Check sheet for the modelled part. Datum: model origin and axes. Units: mm. A direction names the side the tool comes from. Round coordinates to 2 decimals unless told otherwise and drop trailing zeros. Order: outer loops, then holes, each group sorted by start corner. A loop starts at its lowest first (then second) coordinate and runs counter-clockwise, first axis right, second up.
```python
from build123d import *

# Parameters (mm, degrees)
SKETCH_1_R             = 0.5
EXTRUDE_1_DEPTH        = 8
EXTRUDE_2_DEPTH        = 21.5
EXTRUDE_3_DEPTH        = 9
SKETCH_4_R             = 3
EXTRUDE_4_DEPTH        = 10
EXTRUDE_5_DEPTH        = 9
HOLE_WIZARD_M3_1_D     = 2.5
HOLE_WIZARD_M3_1_DEPTH = 6.5
HOLE_WIZARD_M3_1_TIP   = 0.751075774
SKETCH_10_R            = 11
EXTRUDE_6_DEPTH        = 2
SKETCH_11_R            = 4.75
CUT_EXTRUDE_1_DEPTH    = 22
SKETCH_12_W            = 16
SKETCH_12_H            = 4
EXTRUDE_7_DEPTH        = 20
SKETCH_13_W            = 16
SKETCH_13_H            = 5.5
CUT_EXTRUDE_2_DEPTH    = 4
SKETCH_14_W            = 16
SKETCH_14_H            = 0.410991047
CUT_EXTRUDE_3_DEPTH    = 3
SKETCH_15_W            = 14.932119024
SKETCH_15_H            = 4.421120872
SKETCH_15_W_2          = 1.018591574
SKETCH_15_H_2          = 0.888558607
SKETCH_15_W_3          = 0.910230768
SKETCH_15_W_4          = 1.105280218
SKETCH_15_W_5          = 0.95357509
SKETCH_15_W_6          = 1.365346151
SKETCH_15_W_7          = 14.029885449
SKETCH_15_H_3          = 2.651802524
SKETCH_15_W_8          = 0.733211095
SKETCH_15_H_4          = 0.986717219
SKETCH_15_W_9          = 0.549388278
SKETCH_15_W_10         = 0.68897455
SKETCH_15_W_11         = 1.063804501
SKETCH_15_W_12         = 0.745609389
SKETCH_15_W_13         = 0.832542653
CUT_EXTRUDE_4_DEPTH    = 3
SKETCH_16_W            = 3.5
SKETCH_16_H            = 23
EXTRUDE_8_DEPTH        = 5.5
SKETCH_17_W            = 23
SKETCH_17_H            = 3.5
CUT_EXTRUDE_5_DEPTH    = 1
SKETCH_18_W            = 21.377042826
SKETCH_18_H            = 3.957601196
SKETCH_18_W_2          = 1.139309436
SKETCH_18_H_2          = 1.169291262
SKETCH_18_W_3          = 0.929436644
SKETCH_18_W_4          = 1.109327608
SKETCH_18_W_5          = 1.349182226
SKETCH_18_W_6          = 1.259236744
SKETCH_18_W_7          = 1.319200399
CUT_EXTRUDE_6_DEPTH    = 3


with BuildPart() as part:
    # 草图1 → 凸台-拉伸1 (new body)
    with BuildSketch(Plane(origin=(0, 0, 0), x_dir=(1, 0, 0), z_dir=(0, 1, 0))):
        Polygon((-21, 17.5), (-17.5, 21), (17.5, 21), (21, 17.5), (21, -17.5), (17.5, -21), (-17.5, -21), (-21, -17.5), align=None)
        with Locations(Location((-15.5, 15.5, 0), (0, 0, 270))):
            Circle(SKETCH_1_R, mode=Mode.SUBTRACT)
        with Locations(Location((15.5, 15.5, 0), (0, 0, 270))):
            Circle(SKETCH_1_R, mode=Mode.SUBTRACT)
        with Locations(Location((-15.5, -15.5, 0), (0, 0, 270))):
            Circle(SKETCH_1_R, mode=Mode.SUBTRACT)
        with Locations(Location((15.5, -15.5, 0), (0, 0, 270))):
            Circle(SKETCH_1_R, mode=Mode.SUBTRACT)
    extrude(amount=EXTRUDE_1_DEPTH)

    # 草图2 → 凸台-拉伸2 (add)
    with BuildSketch(Plane.XZ):
        with BuildLine():
            Line((-20.414213562, 14.585786438), (-14.585786438, 20.414213562))
            ThreePointArc((-14.585786438, 20.414213562), (-13.93693974, 20.847759065), (-13.171572875, 21))
            Line((-13.171572875, 21), (13.171572875, 21))
            ThreePointArc((13.171572875, 21), (13.93693974, 20.847759065), (14.585786438, 20.414213562))
            Line((14.585786438, 20.414213562), (20.414213562, 14.585786438))
            ThreePointArc((20.414213562, 14.585786438), (20.847759065, 13.93693974), (21, 13.171572875))
            Line((21, 13.171572875), (21, -13.171572875))
            ThreePointArc((21, -13.171572875), (20.847759065, -13.93693974), (20.414213562, -14.585786438))
            Line((20.414213562, -14.585786438), (14.585786438, -20.414213562))
            ThreePointArc((14.585786438, -20.414213562), (13.93693974, -20.847759065), (13.171572875, -21))
            Line((13.171572875, -21), (-13.171572875, -21))
            ThreePointArc((-13.171572875, -21), (-13.93693974, -20.847759065), (-14.585786438, -20.414213562))
            Line((-14.585786438, -20.414213562), (-20.414213562, -14.585786438))
            ThreePointArc((-20.414213562, -14.585786438), (-20.847759065, -13.93693974), (-21, -13.171572875))
            Line((-21, -13.171572875), (-21, 13.171572875))
            ThreePointArc((-21, 13.171572875), (-20.847759065, 13.93693974), (-20.414213562, 14.585786438))
        make_face()
    extrude(amount=EXTRUDE_2_DEPTH)

    # 草图3 → 凸台-拉伸3 (add)
    with BuildSketch(Plane.XZ.offset(21.5)):
        Polygon((-21, 17.5), (-17.5, 21), (17.5, 21), (21, 17.5), (21, -17.5), (17.5, -21), (-17.5, -21), (-21, -17.5), align=None)
    extrude(amount=EXTRUDE_3_DEPTH)

    # 草图4 → 凸台-拉伸4 (add)
    with BuildSketch(Plane.XZ.offset(30.5)):
        with Locations(Location((-15.5, 15.5, 0), (0, 0, 90))):
            Circle(SKETCH_4_R)
        with Locations(Location((15.5, 15.5, 0), (0, 0, 90))):
            Circle(SKETCH_4_R)
        with Locations(Location((-15.5, -15.5, 0), (0, 0, 90))):
            Circle(SKETCH_4_R)
        with Locations(Location((15.5, -15.5, 0), (0, 0, 90))):
            Circle(SKETCH_4_R)
    extrude(amount=EXTRUDE_4_DEPTH)

    # 草图5 → 凸台-拉伸5 (add)
    with BuildSketch(Plane.XZ.offset(40.5)):
        Polygon((-21, 17.5), (-17.5, 21), (17.5, 21), (21, 17.5), (21, -17.5), (17.5, -21), (-17.5, -21), (-21, -17.5), align=None)
    extrude(amount=-EXTRUDE_5_DEPTH)

    # M3 螺纹孔的螺纹孔钻头1
    with Locations(Plane(origin=(0, 8, 0), x_dir=(1, 0, 0), z_dir=(0, 1, 0))):
        with Locations((-15.5, 15.5), (15.5, 15.5), (-15.5, -15.5), (15.5, -15.5)):
            Hole(HOLE_WIZARD_M3_1_D / 2, depth=HOLE_WIZARD_M3_1_DEPTH)
            with Locations((0, 0, -(HOLE_WIZARD_M3_1_DEPTH + HOLE_WIZARD_M3_1_TIP / 2))):  # 118° drill point
                Cone(0, HOLE_WIZARD_M3_1_D / 2, HOLE_WIZARD_M3_1_TIP, mode=Mode.SUBTRACT)

    # 草图10 → 凸台-拉伸6 (add)
    with BuildSketch(Plane(origin=(0, 8, 0), x_dir=(1, 0, 0), z_dir=(0, 1, 0))):
        with Locations(Location((0, 0, 0), (0, 0, 90))):
            Circle(SKETCH_10_R)
    extrude(amount=EXTRUDE_6_DEPTH)

    # 草图11 → 切除-拉伸1 (cut)
    with BuildSketch(Plane(origin=(0, 10, 0), x_dir=(1, 0, 0), z_dir=(0, 1, 0))):
        with Locations(Location((0, 0, 0), (0, 0, 270))):
            Circle(SKETCH_11_R)
    extrude(amount=-CUT_EXTRUDE_1_DEPTH, mode=Mode.SUBTRACT)

    # 草图12 → 凸台-拉伸7 (add)
    with BuildSketch(Plane.XZ.offset(40.5)):
        with Locations((0, 23)):
            Rectangle(SKETCH_12_W, SKETCH_12_H)
    extrude(amount=-EXTRUDE_7_DEPTH)

    # 草图13 → 切除-拉伸2 (cut)
    with BuildSketch(Plane.XY.offset(25)):
        with Locations((0, -33.25)):
            Rectangle(SKETCH_13_W, SKETCH_13_H)
    extrude(amount=-CUT_EXTRUDE_2_DEPTH, mode=Mode.SUBTRACT)

    # 草图14 → 切除-拉伸3 (cut)
    with BuildSketch(Plane.XY.offset(25)):
        with Locations((0, -28.356047823)):
            Rectangle(SKETCH_14_W, SKETCH_14_H)
    extrude(amount=-CUT_EXTRUDE_3_DEPTH, mode=Mode.SUBTRACT)

    # 草图15 → 切除-拉伸4 (cut)
    # profile 1 of 2: a face of its own
    with BuildSketch(Plane.XY.offset(25)):
        with Locations((0.04248549, -23.883266216)):
            Rectangle(SKETCH_15_W, SKETCH_15_H)
        with Locations((-6.090736112, -23.850757974)):
            Rectangle(SKETCH_15_W_2, SKETCH_15_H_2, mode=Mode.SUBTRACT)
        with Locations((-4.172749851, -23.850757974)):
            Rectangle(SKETCH_15_W_3, SKETCH_15_H_2, mode=Mode.SUBTRACT)
        with Locations((-2.092222382, -23.850757974)):
            Rectangle(SKETCH_15_W_3, SKETCH_15_H_2, mode=Mode.SUBTRACT)
        with Locations((0.215862779, -23.850757974)):
            Rectangle(SKETCH_15_W_4, SKETCH_15_H_2, mode=Mode.SUBTRACT)
        with Locations((2.177193362, -23.850757974)):
            Rectangle(SKETCH_15_W_5, SKETCH_15_H_2, mode=Mode.SUBTRACT)
        with Locations((5.027082552, -23.850757974)):
            Rectangle(SKETCH_15_W_6, SKETCH_15_H_2, mode=Mode.SUBTRACT)
    # profile 2 of 2: a face of its own
    with BuildSketch(Plane.XY.offset(25)):
        with Locations((0.146506967, -38.103976676)):
            Rectangle(SKETCH_15_W_7, SKETCH_15_H_3)
        with Locations((-5.724130565, -38.073141763)):
            Rectangle(SKETCH_15_W_8, SKETCH_15_H_4, mode=Mode.SUBTRACT)
        with Locations((-3.442940328, -38.073141763)):
            Rectangle(SKETCH_15_W_9, SKETCH_15_H_4, mode=Mode.SUBTRACT)
        with Locations((-1.292619723, -38.073141763)):
            Rectangle(SKETCH_15_W_10, SKETCH_15_H_4, mode=Mode.SUBTRACT)
        with Locations((0.678409218, -38.073141763)):
            Rectangle(SKETCH_15_W_11, SKETCH_15_H_4, mode=Mode.SUBTRACT)
        with Locations((3.026785602, -38.073141763)):
            Rectangle(SKETCH_15_W_12, SKETCH_15_H_4, mode=Mode.SUBTRACT)
        with Locations((4.98758832, -38.073141763)):
            Rectangle(SKETCH_15_W_13, SKETCH_15_H_4, mode=Mode.SUBTRACT)
    extrude(amount=-CUT_EXTRUDE_4_DEPTH, mode=Mode.SUBTRACT)

    # 草图16 → 凸台-拉伸8 (add)
    with BuildSketch(Plane.XZ.offset(40.5)):
        with Locations((22.75, 0)):
            Rectangle(SKETCH_16_W, SKETCH_16_H)
    extrude(amount=-EXTRUDE_8_DEPTH)

    # 草图17 → 切除-拉伸5 (cut)
    with BuildSketch(Plane(origin=(21, 0, 0), x_dir=(0, 0, -1), z_dir=(1, 0, 0))):
        with Locations((0, -33.25)):
            Rectangle(SKETCH_17_W, SKETCH_17_H)
    extrude(amount=-CUT_EXTRUDE_5_DEPTH, mode=Mode.SUBTRACT)

    # 草图18 → 切除-拉伸6 (cut)
    with BuildSketch(Plane(origin=(24.5, 0, 0), x_dir=(0, 0, -1), z_dir=(1, 0, 0))):
        with Locations((-0.141025196, -37.937429966)):
            Rectangle(SKETCH_18_W, SKETCH_18_H)
        with Locations((-8.790782356, -38.102330016)):
            Rectangle(SKETCH_18_W_2, SKETCH_18_H_2, mode=Mode.SUBTRACT)
        with Locations((-4.938117555, -38.102330016)):
            Rectangle(SKETCH_18_W_3, SKETCH_18_H_2, mode=Mode.SUBTRACT)
        with Locations((-1.640116558, -38.102330016)):
            Rectangle(SKETCH_18_W_4, SKETCH_18_H_2, mode=Mode.SUBTRACT)
        with Locations((1.268120685, -38.102330016)):
            Rectangle(SKETCH_18_W_5, SKETCH_18_H_2, mode=Mode.SUBTRACT)
        with Locations((3.951494223, -38.102330016)):
            Rectangle(SKETCH_18_W_6, SKETCH_18_H_2, mode=Mode.SUBTRACT)
        with Locations((8.029022729, -38.102330016)):
            Rectangle(SKETCH_18_W_7, SKETCH_18_H_2, mode=Mode.SUBTRACT)
    extrude(amount=-CUT_EXTRUDE_6_DEPTH, mode=Mode.SUBTRACT)


solid = part.part
```
Item 1: Go/stop test with flat-tipped pins: P1, Ø2, axis at x = -10, z = 16.5, coming from the +Y side; P2, Ø0.9, axis at x = 23.5, y = -37.5, coming from the +Z side; P3, Ø2, axis at x = 15.5, z = 15.5, coming from the +Y side. Record where each tip stops, or that it passes through.
Answer:
P1: stops at y = 8
P2: stops at z = 11.5
P3: stops at y = 1.35
Item 2: Sectioned sample at B-B (y = -15). Record the cut outline in (x, z), and give its area (3 significant figures).
Answer:
outline: (-21, -13.17) arc R2 ccw to (-20.41, -14.59) - (-14.59, -20.41) arc R2 ccw to (-13.17, -21) - (13.17, -21) arc R2 ccw to (14.59, -20.41) - (20.41, -14.59) arc R2 ccw to (21, -13.17) - (21, 13.17) arc R2 ccw to (20.41, 14.59) - (14.59, 20.41) arc R2 ccw to (13.17, 21) - (-13.17, 21) arc R2 ccw to (-14.59, 20.41) - (-20.41, 14.59) arc R2 ccw to (-21, 13.17) - close
area: 1,670 mm2
Item 3: Sectioned sample at A-A (y = -3). Record the cut outline in (x, z), and give its area (3 significant figures).
Answer:
outline: (-21, -13.17) arc R2 ccw to (-20.41, -14.59) - (-14.59, -20.41) arc R2 ccw to (-13.17, -21) - (13.17, -21) arc R2 ccw to (14.59, -20.41) - (20.41, -14.59) arc R2 ccw to (21, -13.17) - (21, 13.17) arc R2 ccw to (20.41, 14.59) - (14.59, 20.41) arc R2 ccw to (13.17, 21) - (-13.17, 21) arc R2 ccw to (-14.59, 20.41) - (-20.41, 14.59) arc R2 ccw to (-21, 13.17) - close; hole circle Ø9.5 at (0, 0)
area: 1,590 mm2
Item 4: Sectioned sample at C-C (y = -32.5). Record the cut outline in (x, z).
Answer:
outline: (-21, -17.5) - (-17.5, -21) - (17.5, -21) - (21, -17.5) - (21, -11.5) - (20, -11.5) - (20, 11.5) - (21, 11.5) - (21, 17.5) - (17.5, 21) - (-17.5, 21) - (-21, 17.5) - close
Item 5: Scan lines: line 1 along X through (y, z) = (5.25, -15.5); line 2 along Y through (x, z) = (-12, 13). Record each from-to range of solid material in increasing order.
Answer:
line 1: x = -21 to -16.75, -14.25 to 14.25, 16.75 to 21
line 2: y = -40.5 to -31.5, -30.5 to 8
Item 6: Access from +Z, -Z, +X, -X, +Y, -Y to the whole of each face (thin tool, end or side, straight path). Record for faces 4 (the flat face through (7.161, -38, 24)), 5 (the flat face through (19, 0, 18)), 6 (the cylindrical face through (-13.93, -10.6, -20.85)), 7 (the cylindrical face through (16.421, 4.704, -16.345)).
Answer:
face 4: +Z
face 5: +Z, +X
face 6: -Z, -X
face 7: +Y
Item 7: Release check for a two-part mould opening along Y. For faces 1 (the flat face through (23, -38, 10.83)), 2 (the flat face through (1, -40.5, 2)), 3 (the flat face through (-8, -26, 23)) record: released by +Y, released by -Y, zero draft, split by the parting line, or undercut.
Answer:
face 1: undercut
face 2: released by -Y
face 3: zero draft
